```python
from build123d import *

# Parameters (mm, degrees)
BOSS_EXTRUDE1_DEPTH      = 20
BOSS_EXTRUDE1_DEPTH_BACK = 20
CUT_EXTRUDE1_DEPTH       = 32.020154738
CUT_EXTRUDE1_DEPTH_BACK  = 32.020154738


with BuildPart() as part:
    # Sketch1 → Boss-Extrude1 (new, two sides: drawn at the far end of the back side and taken through both)
    with BuildSketch(Plane(origin=(0, 0, 0), x_dir=(0, 0, -1), z_dir=(1, 0, 0)).offset(-BOSS_EXTRUDE1_DEPTH_BACK)):
        Polygon((-16, 17.5), (5, 17.5), (5, -17.5), (-5, -17.5), (-5, 10.5), (-16, 10.5), align=None)
    extrude(amount=BOSS_EXTRUDE1_DEPTH + BOSS_EXTRUDE1_DEPTH_BACK)

    # Sketch2 → Cut-Extrude1 (cut, two sides: drawn at the far end of the back side and taken through both)
    with BuildSketch(Plane.XY.offset(-CUT_EXTRUDE1_DEPTH_BACK)):
        with BuildLine():
            ThreePointArc((-5, -2.5), (-6.464466094, 1.035533906), (-10, 2.5))
            ThreePointArc((-10, 2.5), (-13.535533906, 1.035533906), (-15, -2.5))
            Line((-15, -2.5), (-5, -2.5))
        make_face()
        with BuildLine():
            ThreePointArc((-10, -7.5), (-6.464466094, -6.035533906), (-5, -2.5))
            Line((-5, -2.5), (-15, -2.5))
            ThreePointArc((-15, -2.5), (-13.535533906, -6.035533906), (-10, -7.5))
        make_face()
        with BuildLine():
            Line((20, 2.5), (-10, 2.5))
            ThreePointArc((-10, 2.5), (-6.464466094, 1.035533906), (-5, -2.5))
            Line((-5, -2.5), (20, -2.5))
            Line((20, -2.5), (20, 2.5))
        make_face()
        with BuildLine():
            Line((20, -2.5), (-5, -2.5))
            ThreePointArc((-5, -2.5), (-6.464466094, -6.035533906), (-10, -7.5))
            Line((-10, -7.5), (20, -7.5))
            Line((20, -7.5), (20, -2.5))
        make_face()
    extrude(amount=CUT_EXTRUDE1_DEPTH + CUT_EXTRUDE1_DEPTH_BACK, mode=Mode.SUBTRACT)


solid = part.part
```
Geometry check sheet. Reference: the model listing, model coordinates, mm. A direction names the side the tool comes from. Give positions to 0.01 mm unless a question says otherwise; leave off trailing zeros. Order: outer loops, then holes, each group sorted by start corner. A loop starts at its lowest first (then second) coordinate and runs counter-clockwise, first axis right, second up.
1. Thickness scan on L1, parallel to Y at x = 11.5, z = -1.5; L2, parallel to Y at x = -0.5, z = 11.5; L3, parallel to Z at x = -5.5, y = -11. Record the ranges inside material, lowest first.
2. Gauge pin test, flat ends, axial feed: pin 1 Ø8 at (x, y) = (3.5, 2.5) entering from +Z; pin 2 Ø3.5 at (x, z) = (4, 12) entering from -Y; pin 3 Ø12 at (x, y) = (4.5, -1.5) entering from -Z; pin 4 Ø5 at (x, y) = (7.5, -1.5) entering from +Z. Record the tip position at first contact, or that the pin passes through.
3. Section check C-C, the plane y = -15. Enter the section's corners in (x, z), and give its area (3 significant figures).
4. Section check A-A, the plane x = 10.5. Enter the section's corners in (y, z), and give its area (3 significant figures).
5. Access from +Z, -Z, +X, -X, +Y, -Y to the whole of each face (thin tool, end or side, straight path). Record for faces 1 (the face through (0, 10.5, 10)), 2 (the face through (5, -7.5, 0)), 3 (the face through (0, 14, 16)).
6. Section check B-B, the plane z = -1.75. Enter the section's corners in (x, y).
7. Section check D-D, the plane z = 9.25. Enter the section's corners in (x, y).
Values follow:
1. L1: y = -17.5 to -7.5, 2.5 to 17.5
1. L2: y = 10.5 to 17.5
1. L3: z = -5 to 5
2. pin 1: stops at z = 5
2. pin 2: stops at y = 10.5
2. pin 3: stops at z = -5
2. pin 4: passes through
3. outline: (-20, -5) - (20, -5) - (20, 5) - (-20, 5) - close
3. area: 400 mm2
4. outline: (-17.5, -5) - (-7.5, -5) - (-7.5, 5) - (-17.5, 5) - close; (2.5, -5) - (17.5, -5) - (17.5, 16) - (10.5, 16) - (10.5, 5) - (2.5, 5) - close
4. area: 327 mm2
5. face 1: +Z, +X, -X, -Y
5. face 2: +Z, -Z, +X
5. face 3: +Z, +X, -X, +Y, -Y
6. outline: (-20, -17.5) - (20, -17.5) - (20, -7.5) - (-10, -7.5) arc R5 cw to (-10, 2.5) - (20, 2.5) - (20, 17.5) - (-20, 17.5) - close
7. outline: (-20, 10.5) - (20, 10.5) - (20, 17.5) - (-20, 17.5) - close
